Autodesk Inventor part; units mm, degrees
ref_plane "YZ Plane" through (0, 0, 0) normal (1, 0, 0) x (0, 1, 0)
ref_plane "XZ Plane" through (0, 0, 0) normal (0, 1, 0) x (-1, 0, 0)
ref_plane "XY Plane" through (0, 0, 0) normal (0, 0, 1) x (1, 0, 0)
sketch "Boceto1" plane through (0, 0, 0) normal (0, 1, 0) x (-1, 0, 0)
  line L0 (25.5, 15) -> (-25.5, 15)
  line L1 (-25.5, 15) -> (-25.5, -15)
  line L2 (-25.5, -15) -> (25.5, -15)
  line L3 (25.5, -15) -> (25.5, 15)
  line L4 (25.5, 15) -> (-25.5, -15) construction
  line L5 (-25.5, 15) -> (25.5, -15) construction
  line L6 (-15.5, 15) -> (-15.5, -15)
  line L7 (0, 15) -> (0, 11.847)
  line L8 (-25.5, 0) -> (-22.3332, 0)
  line L9 (25.5, 15) -> (25.5, -15)
  line L10 (15.5, 15) -> (15.5, -15)
  line L11 (25.5, 0) -> (22.3332, 0)
  line L12 (-25.5, -15) -> (-25.5, 15)
  line L13 (-25.5, 0) -> (-22.3332, 0)
  line L14 (-25.5, 15) -> (-25.5, -15)
  point P0 (0, 0)
  point P1 (31.5, 22.5)
  dimension "d2" = 10
  dimension "d21" = 51
  dimension "d22" = 30
extrude "Extrusión1" add sketch "Boceto1" along normal blind 5 contours L3 L2 L10 L0 | L6 L2 L1 L0
sketch "Boceto4" plane through (0, 0, 0) normal (0, 1, 0) x (-1, 0, 0)
  line L0 (-28.5, 18) -> (28.5, 18)
  line L1 (28.5, 18) -> (28.5, -18)
  line L2 (28.5, -18) -> (-28.5, -18)
  line L3 (-28.5, -18) -> (-28.5, 18)
  line L4 (-28.5, 18) -> (28.5, -18) construction
  line L5 (28.5, 18) -> (-28.5, -18) construction
  line L6 (28.5, -15) -> (-28.5, -15)
  line L7 (-28.5, 15) -> (28.5, 15)
  line L8 (25.5, -18) -> (25.5, 18)
  line L9 (-25.5, 18) -> (-25.5, -18)
  line L10 (-25.5, -15) -> (-15.5, -15)
  point P0 (0, 0)
  point P1 (-25.5, -15)
  point P2 (-25.5, 15)
  point P3 (25.5, 15)
  point P4 (25.5, -15)
  dimension "d23" = 57
  dimension "d24" = 36
  dimension "d27" = 0
extrude "Extrusión4" add sketch "Boceto4" along normal blind 5 contours L0 L8 L7 L9 | L7 L9 L6 L3 | L7 L1 L6 L8 | L6 L8 L2 L9
sketch "Boceto5" plane through (0, 5, 0) normal (0, 1, 0) x (1, 0, 0)
  line L0 (25.5, 18) -> (-25.5, 18)
  line L1 (25.5, 15) -> (25.5, 18)
  line L2 (-25.5, 18) -> (25.5, 18)
  line L3 (25.5, 18) -> (25.5, 15)
  line L4 (25.5, 15) -> (-25.5, 15)
  line L5 (-25.5, 15) -> (-25.5, 18)
  point P0 (0, 0)
extrude "Extrusión5" add sketch "Boceto5" along normal blind 49
sketch "Boceto6" plane through (-15.5, 0, -15) normal (0, 0, 1) x (1, 0, 0)
  circle A0 centre (32, 45) radius 2
  line L0 (41, 5) -> (41, 54)
  line L1 (-10, 54) -> (41, 54)
  line L2 (-10, 5) -> (-10, 54)
  line L3 (-10, 29.5) -> (15.5, 29.5)
  line L4 (15.5, 29.5) -> (15.5, 54)
  circle A1 centre (0, 46) radius 2
  circle A2 centre (-1, 14) radius 2
  circle A3 centre (31, 13) radius 2
  point P0 (15.5, 0)
  dimension "d30" = 4
  dimension "d31" = 9
  dimension "d32" = 9
  dimension "d35" = 360
extrude "Extrusión6" cut sketch "Boceto6" against normal blind 49 contours A0 | A1 | A2 | A3
sketch "Boceto7" plane through (0, 5, 0) normal (0, 1, 0) x (1, 0, 0)
  line L0 (-28.5, 15) -> (-28.5, -15)
  line L1 (-28.5, 15) -> (-25.5, 15)
  line L2 (-25.5, 15) -> (-25.5, -15)
  line L3 (-25.5, -15) -> (-28.5, -15)
  line L4 (-28.5, -15) -> (-28.5, 15)
  line L5 (28.5, 15) -> (25.5, 15)
  line L6 (25.5, -15) -> (28.5, -15)
  line L7 (28.5, 15) -> (25.5, 15)
  line L8 (25.5, 15) -> (25.5, -15)
  line L9 (25.5, -15) -> (28.5, -15)
  line L10 (28.5, -15) -> (28.5, 15)
  point P0 (0, 0)
  point P1 (25.5, -18)
extrude "Extrusión7" add sketch "Boceto7" along normal blind 49
sketch "Boceto12" plane through (0, 0, 0) normal (0, -1, 0) x (1, 0, 0)
  line L0 (-35, -35) -> (35, -35)
  line L1 (35, -35) -> (35, 35)
  line L2 (35, 35) -> (-35, 35)
  line L3 (-35, 35) -> (-35, -35)
  line L4 (-35, -35) -> (35, 35) construction
  line L5 (35, -35) -> (-35, 35) construction
  line L6 (30, 30) -> (-30, 30)
  line L7 (-30, 30) -> (-30, -30)
  line L8 (-30, -30) -> (30, -30)
  line L9 (30, -30) -> (30, 30)
  line L10 (30, 30) -> (-30, -30) construction
  line L11 (-30, 30) -> (30, -30) construction
  circle A0 centre (-30, 30) radius 2.6
  circle A1 centre (30, 30) radius 2.6
  circle A2 centre (30, -30) radius 2.6
  circle A3 centre (-30, -30) radius 2.6
  line L12 (15.5, -15) -> (15.5, 15)
  line L13 (-15.5, -15) -> (15.5, -15)
  line L14 (15.5, -15) -> (15.5, 15)
  line L15 (15.5, 15) -> (-15.5, 15)
  line L16 (-15.5, 15) -> (-15.5, -15)
  line L17 (-15.5, -15) -> (15.5, 15) construction
  line L18 (15.5, -15) -> (-15.5, 15) construction
  point P0 (0, 0)
  point P1 (0, 0)
  dimension "d63" = 70
  dimension "d64" = 70
  dimension "d65" = 60
  dimension "d66" = 5.2
  dimension "d67" = 5.2
  dimension "d68" = 5.2
  dimension "d69" = 5.2
extrude "Extrusión10" add sketch "Boceto12" against normal blind 5 contours L3 L2 L1 L0 | L6 A1 L9 A2 L8 A3 L7 A0
properties part number "depth_camera_fastening"
Design review of the part built by this model. Coordinates are the model's own, in mm. A direction names the side the tool comes from. Coordinates: 2 decimals unless noted, no trailing zeros. Order: outer loops, then holes, each group sorted by start corner. A loop starts at its lowest first (then second) coordinate and runs counter-clockwise, first axis right, second up.
1) Take a section at A-A, the plane x = -30. Give the boundary of the cut face in (y, z), and give its area (3 significant figures).
2) Mouldability with a two-part tool opening along Y and no side actions: class faces 5 (the cylindrical face through (16.066, 43.048, -16.479)), 6 (the flat face through (-25.5, 29, -16)), 7 (the flat face through (-27, 54, 0)) as +Y half, -Y half, draft (parallel to the pull), parting line (faces both ways), or undercut.
3) Take a section at C-C, the plane z = 4. Give the boundary of the cut face in (x, y), and give its area (3 significant figures).
4) Wall thickness on line 1 along X through (y, z) = (3.8, -30); line 2 along X through (y, z) = (25, 11.5): over which ranges is each line inside the solid? List them lowest first.
5) Clearance check with flat-ended pins moving along their axes: pin 1 (6 mm diameter, centred on y = 10.5, z = 15, fed in from +X); pin 2 (5 mm diameter, centred on x = -15.5, y = 46, fed in from +Z); pin 3 (9 mm diameter, centred on y = 40, z = -2.5, fed in from -X). State where each tip first meets the part, or that it passes through.
6) For faces 1 (the flat face through (-27, 29, 15)), 2 (the flat face through (0, 29, -18)), 3 (the flat face through (0, 2, 15)), 4 (the flat face through (-25.5, 29, 0)), list the 3-axis set-ups (+Z, -Z, +X, -X, +Y, -Y) from which the entire face can be reached by the end or side of a thin tool; tool diameter is ignored.
7) Take a section at D-D, the plane x = 6.5. Give the boundary of the cut face in (y, z).
Returned:
1. outline: (0, -35) - (5, -35) - (5, -32.6) - (0, -32.6) - close; (0, -27.4) - (5, -27.4) - (5, 27.4) - (0, 27.4) - close; (0, 32.6) - (5, 32.6) - (5, 35) - (0, 35) - close
1. area: 298 mm2
2. face 5: undercut
2. face 6: draft
2. face 7: +Y half
3. outline: (-35, 0) - (-15.5, 0) - (-15.5, 5) - (-25.5, 5) - (-25.5, 54) - (-28.5, 54) - (-28.5, 5) - (-35, 5) - close; (15.5, 0) - (35, 0) - (35, 5) - (28.5, 5) - (28.5, 54) - (25.5, 54) - (25.5, 5) - (15.5, 5) - close
3. area: 489 mm2
4. line 1: x = -35 to -32.6, -27.4 to 27.4, 32.6 to 35
4. line 2: x = -28.5 to -25.5, 25.5 to 28.5
5. pin 1: stops at x = 28.5
5. pin 2: stops at z = -15
5. pin 3: stops at x = -28.5
6. face 1: +Z, +X, -X, +Y
6. face 2: -Z, +X, -X, +Y
6. face 3: +Y, -Y
6. face 4: +Z, +Y
7. outline: (0, -35) - (5, -35) - (5, -18) - (54, -18) - (54, -15) - (0, -15) - close; (0, 15) - (5, 15) - (5, 35) - (0, 35) - close
